```python
from build123d import *

# Parameters (mm, degrees)
F0_W     = 200
F0_H     = 45
F1_DEPTH = 9
F2_W     = 4.5
F2_H     = 4.5
F3_DEPTH = 200.001
F4_W     = 4.5
F4_H     = 4.5
F5_DEPTH = 40.501


with BuildPart() as f1:
    # F0 (on Right) → F1 (new body)
    with BuildSketch(Plane.YZ):
        Rectangle(F0_W, F0_H)
    extrude(amount=F1_DEPTH)

    # F2 (on face) → F3 (cut, through all)
    with BuildSketch(Plane.XZ.offset(100)):
        with Locations((2.25, 20.25)):
            Rectangle(F2_W, F2_H)
    extrude(amount=-F3_DEPTH, mode=Mode.SUBTRACT)

    # F4 (on face) → F5 (cut, through all)
    with BuildSketch(Plane.XY.offset(18)):
        with Locations((2.25, -97.75)):
            Rectangle(F4_W, F4_H)
    extrude(amount=-F5_DEPTH, mode=Mode.SUBTRACT)


solid = f1.part
```
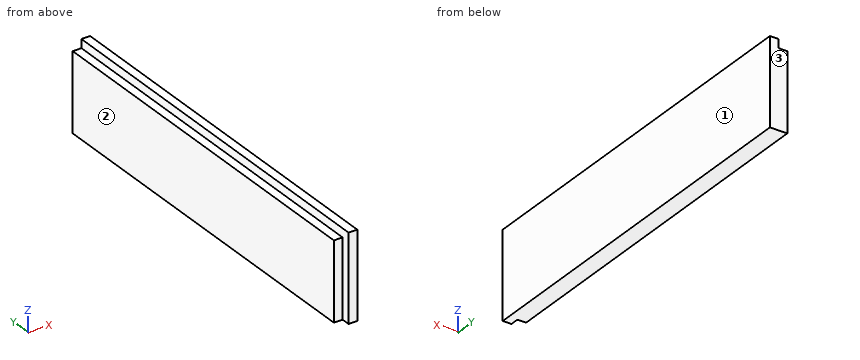
Input: part model. Units: mm. Frame: model coordinates. Face numbers are marked on the shaded views. Round coordinates to 2 decimals unless told otherwise and drop trailing zeros. Loops run counter-clockwise (first coordinate to the right, second up) from the corner with the lowest first, then second, coordinate; pieces in that order, holes last. Notation, with made-up numbers: M 4,26.5 L 45,26.5 A17 cw 45,37.5 Z; hole C 7.5,14 d6. An arc over 180 degrees is marked long. Answer in a Markdown table with one row per item. Add a question column.
1. Ray query, probe 1 along Z at (x, y) = (1, -35); probe 2 along Y at (x, z) = (3, 14.5). Return the intervals inside material, ascending.
2. Section B-B (y = -57.5). Output: boundary loops of the cut face in (x, z).
3. Contact query for flat-ended pins moving along their axis: pin 1 (3.5 mm diameter, centred on x = 2.5, y = -20.5, fed in from +Z); pin 2 (1 mm diameter, centred on x = 2.5, z = 7, fed in from -Y). Output: stop coordinate, or through.
4. Mould query, pull axis X, two halves, no side actions, for the marked faces 1, 2 and 3. Classes: released by +X, released by -X, zero draft, split by the parting line, or undercut.
5. Section A-A (x = 2.5). Output: boundary loops of the cut face in (y, z).
Values follow:
| question | item | result |
|---|---|---|
| 1 | probe 1 | -22.5 to 18 |
| 1 | probe 2 | -95.5 to 100 |
| 2 | outline | M 0,-22.5 L 9,-22.5 L 9,22.5 L 4.5,22.5 L 4.5,18 L 0,18 Z |
| 3 | pin 1 | z = 18 |
| 3 | pin 2 | y = -95.5 |
| 4 | face 1 | released by +X |
| 4 | face 2 | released by -X |
| 4 | face 3 | zero draft |
| 5 | outline | M -95.5,-22.5 L 100,-22.5 L 100,18 L -95.5,18 Z |
